from build123d import *

# Parameters (mm, degrees)
SKETCH1_R           = 67.5
BOSS_EXTRUDE1_DEPTH = 15
SKETCH2_R           = 47.25
SKETCH2_R_2         = 25
CUT_EXTRUDE1_DEPTH  = 6
SKETCH3_R           = 10
CUT_EXTRUDE2_DEPTH  = 10
SKETCH5_R           = 2.5
CUT_EXTRUDE3_DEPTH  = 10
SKETCH6_R           = 2
CUT_EXTRUDE4_DEPTH  = 15
SKETCH7_R           = 5
CUT_EXTRUDE5_DEPTH  = 5


with BuildPart() as part:
    # Sketch1 → Boss-Extrude1 (new body)
    with BuildSketch(Plane(origin=(0, 0, 0), x_dir=(1, 0, 0), z_dir=(0, 1, 0))):
        Circle(SKETCH1_R)
    extrude(amount=BOSS_EXTRUDE1_DEPTH)

    # Sketch2 → Cut-Extrude1 (cut)
    with BuildSketch(Plane(origin=(0, 15, 0), x_dir=(1, 0, 0), z_dir=(0, 1, 0))):
        Circle(SKETCH2_R)
        Circle(SKETCH2_R_2, mode=Mode.SUBTRACT)
    extrude(amount=-CUT_EXTRUDE1_DEPTH, mode=Mode.SUBTRACT)

    # Sketch3 → Cut-Extrude2 (cut)
    with BuildSketch(Plane(origin=(0, 15, 0), x_dir=(1, 0, 0), z_dir=(0, 1, 0))):
        Circle(SKETCH3_R)
    extrude(amount=-CUT_EXTRUDE2_DEPTH, mode=Mode.SUBTRACT)

    # Sketch5 → Cut-Extrude3 (cut)
    with BuildSketch(Plane(origin=(0, 5, 0), x_dir=(1, 0, 0), z_dir=(0, 1, 0))):
        Circle(SKETCH5_R)
    extrude(amount=-CUT_EXTRUDE3_DEPTH, mode=Mode.SUBTRACT)

    # Sketch6 → Cut-Extrude4 (cut)
    with BuildSketch(Plane(origin=(0, 15, 0), x_dir=(1, 0, 0), z_dir=(0, 1, 0))):
        with Locations((0, 57.5)):
            Circle(SKETCH6_R)
        with Locations((49.796460718, 28.75)):
            Circle(SKETCH6_R)
        with Locations((49.796460718, -28.75)):
            Circle(SKETCH6_R)
        with Locations((0, -57.5)):
            Circle(SKETCH6_R)
        with Locations((-49.796460718, -28.75)):
            Circle(SKETCH6_R)
        with Locations((-49.796460718, 28.75)):
            Circle(SKETCH6_R)
    extrude(amount=-CUT_EXTRUDE4_DEPTH, mode=Mode.SUBTRACT)

    # Sketch7 → Cut-Extrude5 (cut)
    with BuildSketch(Plane(origin=(0, 15, 0), x_dir=(1, 0, 0), z_dir=(0, 1, 0))):
        with Locations((0, 57.5)):
            Circle(SKETCH7_R)
        with Locations((49.796460718, 28.75)):
            Circle(SKETCH7_R)
        with Locations((49.796460718, -28.75)):
            Circle(SKETCH7_R)
        with Locations((0, -57.5)):
            Circle(SKETCH7_R)
        with Locations((-49.796460718, -28.75)):
            Circle(SKETCH7_R)
        with Locations((-49.796460718, 28.75)):
            Circle(SKETCH7_R)
    extrude(amount=-CUT_EXTRUDE5_DEPTH, mode=Mode.SUBTRACT)


solid = part.part
The model under review builds one solid part; all positions refer to its coordinate system, in mm. A direction names the side the tool comes from. Round coordinates to 2 decimals unless told otherwise and drop trailing zeros. Loops run counter-clockwise (first coordinate to the right, second up) from the corner with the lowest first, then second, coordinate; pieces in that order, holes last. Notation, with made-up numbers: (36.5, -38) -> (47.5, -38) arc R16 cw to (47.5, -34) -> close; hole circle Ø9 at (16, 2). An arc over 180 degrees is marked (long way). Return JSON: item names as keys, results as strings.
(1) Add section D-D on z = -28.75. Write out the cut boundary in (x, y).
Solved:
{"outline": "(-61.07, 0) -> (-51.8, 0) -> (-51.8, 10) -> (-54.8, 10) -> (-54.8, 15) -> (-61.07, 15) -> close; (-47.8, 0) -> (47.8, 0) -> (47.8, 10) -> (44.8, 10) -> (44.8, 15) -> (37.5, 15) -> (37.5, 9) -> (-37.5, 9) -> (-37.5, 15) -> (-44.8, 15) -> (-44.8, 10) -> (-47.8, 10) -> close; (51.8, 0) -> (61.07, 0) -> (61.07, 15) -> (54.8, 15) -> (54.8, 10) -> (51.8, 10) -> close"}
(2) Add section A-A on z = 0. Write out the cut boundary in (x, y), plus the area to 3 significant figures.
Solved:
{"outline": "(-67.5, 0) -> (-2.5, 0) -> (-2.5, 5) -> (-10, 5) -> (-10, 15) -> (-25, 15) -> (-25, 9) -> (-47.25, 9) -> (-47.25, 15) -> (-67.5, 15) -> close; (2.5, 0) -> (67.5, 0) -> (67.5, 15) -> (47.25, 15) -> (47.25, 9) -> (25, 9) -> (25, 15) -> (10, 15) -> (10, 5) -> (2.5, 5) -> close", "area": "1,530 mm2"}
(3) For pin 1 (18 mm diameter, centred on x = 0, z = 0, fed in from +Y); pin 2 (9 mm diameter, centred on x = -49.8, z = -28.75, fed in from -Y); pin 3 (3 mm diameter, centred on x = -30.5, y = 7, fed in from -Z); pin 4 (4 mm diameter, centred on y = 10, z = -44, fed in from +X), all flat-tipped, find the tip position at first contact; note any pin that passes through.
Solved:
{"pin 1": "y = 5", "pin 2": "y = 0", "pin 3": "z = -60.95", "pin 4": "x = 52.84"}
(4) For line 1 (X direction, y = 11.45, z = -28.75); line 2 (X direction, y = 13.25, z = 0); line 3 (Z direction, x = 51.5, y = 6.5), list the stretches that pass through material, from the lowest coordinate up.
Solved:
{"line 1": "-61.07 to -54.8, -44.8 to -37.5, 37.5 to 44.8, 54.8 to 61.07", "line 2": "-67.5 to -47.25, -25 to -10, 10 to 25, 47.25 to 67.5", "line 3": "-43.63 to -29.8, -27.7 to 27.7, 29.8 to 43.63"}
(5) The part is to be moulded in two halves that separate along X. For faces 1 (the flat face through (0, 15, 11)), 2 (the cylindrical face through (54.4, 12.5, 30.7)), 3 (the cylindrical face through (-53.57, 7.4, 41.07)), say which applies: released by +X, released by -X, zero draft, split by the parting line, or undercut.
Solved:
{"face 1": "zero draft", "face 2": "undercut", "face 3": "split by the parting line"}
(6) Add section B-B on y = 13. State how many separate pieces and enclosed holes the cut face has, plus the area to 3 significant figures.
Solved:
{"separate pieces": "2", "enclosed holes": "8", "area": "8,480 mm2"}
(7) For faces 4 (the cylindrical face through (-0.651, 12.535, 52.543)), 5 (the flat face through (-15, 15, -45)), list the 3-axis set-ups (+Z, -Z, +X, -X, +Y, -Y) from which the entire face can be reached by the end or side of a thin tool; tool diameter is ignored.
Solved:
{"face 4": "+Y", "face 5": "+Z, -Z, +X, -X, +Y"}
